Design review of the part shown in the three views and the two pictorial views. Dimensions are in mm from the part's minimum x, y and z. Round coordinates to 2 decimals unless told otherwise and drop trailing zeros. Loops run counter-clockwise (first coordinate to the right, second up) from the corner with the lowest first, then second, coordinate; pieces in that order, holes last. Notation, with made-up numbers: (88.5, -10.5) -> (103.5, -10.5) arc R21 cw to (103.5, 8.5) -> close; hole circle Ø11 at (-28.5, -21). An arc over 180 degrees is marked (long way). Write each question's results on one line, items separated by ' | '. Start each with the question number.
Item 1: We need section B-B (x = 145). Give the boundary of the cut face in (y, z).
Item 2: Clearance check with flat-ended pins moving along their axes: pin 1 Ø1.5 at (y, z) = (2, 130.5) entering from -X; pin 2 Ø1.5 at (y, z) = (1.5, 66.5) entering from +X; pin 3 Ø1.5 at (y, z) = (2, 1) entering from -X. State where each tip first meets the part, or that it passes through.
Item 3: We need section D-D (z = 63). Give the boundary of the cut face in (x, y), and give its area (3 significant figures).
Item 4: We need section C-C (z = 105.5). Give the boundary of the cut face in (x, y), and give its area (3 significant figures).
Item 5: We need section A-A (y = 2). Give the boundary of the cut face in (x, z).
Item 6: For L1, parallel to X at y = 2.95, z = 105; L2, parallel to Z at x = 136.5, y = 1.7; L3, parallel to X at y = 0.7, z = 134.5, list the stretches that pass through material, from the lowest coordinate up. Write a range as from..to.
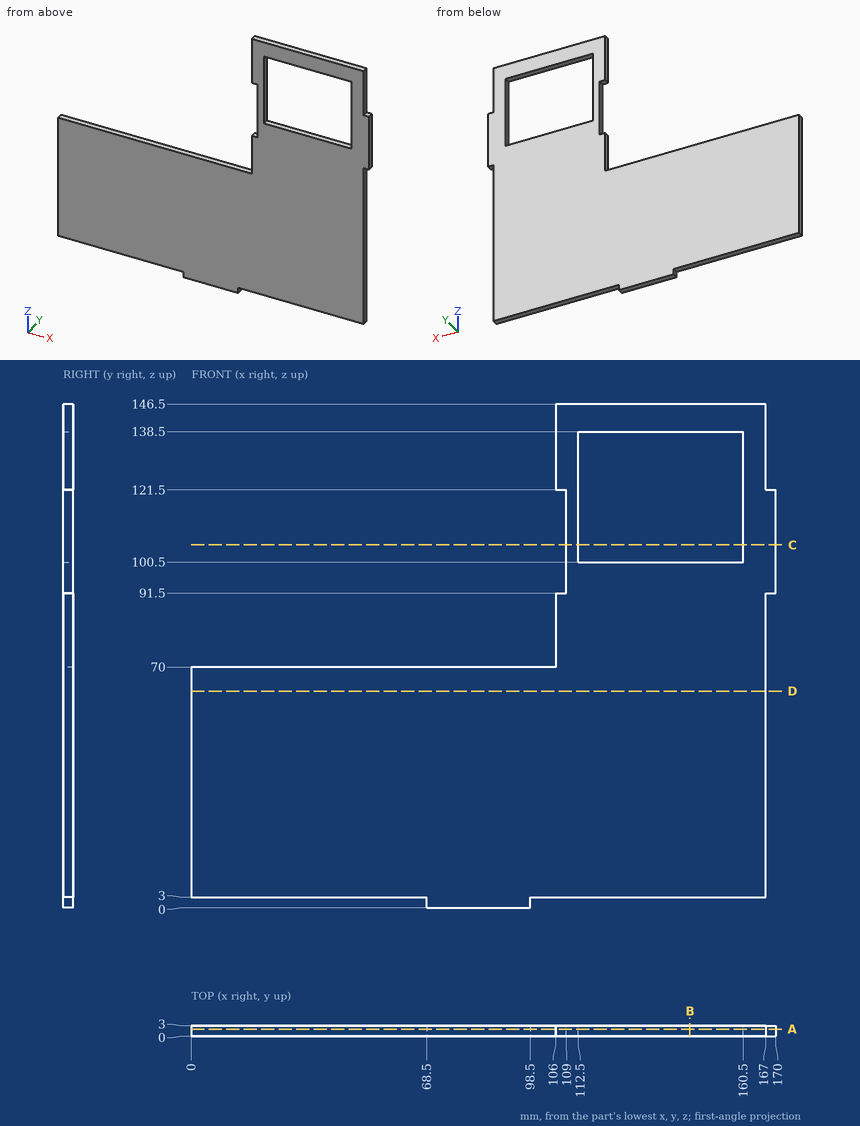
Here are the results:
1) outline: (0, 3) -> (3, 3) -> (3, 100.5) -> (0, 100.5) -> close; (0, 138.5) -> (3, 138.5) -> (3, 146.5) -> (0, 146.5) -> close
2) pin 1: stops at x = 106 | pin 2: stops at x = 167 | pin 3: stops at x = 68.5
3) outline: (0, 0) -> (167, 0) -> (167, 3) -> (0, 3) -> close | area: 501 mm2
4) outline: (109, 0) -> (112.5, 0) -> (112.5, 3) -> (109, 3) -> close; (160.5, 0) -> (170, 0) -> (170, 3) -> (160.5, 3) -> close | area: 39.0 mm2
5) outline: (0, 3) -> (68.5, 3) -> (68.5, 0) -> (98.5, 0) -> (98.5, 3) -> (167, 3) -> (167, 91.5) -> (170, 91.5) -> (170, 121.5) -> (167, 121.5) -> (167, 146.5) -> (106, 146.5) -> (106, 121.5) -> (109, 121.5) -> (109, 91.5) -> (106, 91.5) -> (106, 70) -> (0, 70) -> close; hole (112.5, 100.5) -> (160.5, 100.5) -> (160.5, 138.5) -> (112.5, 138.5) -> close
6) L1: x = 109..112.5, 160.5..170 | L2: z = 3..100.5, 138.5..146.5 | L3: x = 106..112.5, 160.5..167
